```python
from build123d import *

# Parameters (mm, degrees)
SKETCH1_W           = 15.24
SKETCH1_H           = 44.45
SKETCH1_R           = 2.0193
SKETCH1_R_2         = 1.5
BOSS_EXTRUDE1_DEPTH = 3.429
FILLET1_R           = 2.54


with BuildPart() as part:
    # Sketch1 → Boss-Extrude1 (new body)
    with BuildSketch(Plane.XY):
        with Locations((0, 22.225)):
            Rectangle(SKETCH1_W, SKETCH1_H)
        with Locations((0, 4.445)):
            Circle(SKETCH1_R, mode=Mode.SUBTRACT)
        with Locations((0, 16.51)):
            Circle(SKETCH1_R, mode=Mode.SUBTRACT)
        with Locations((-5.08, 42.291)):
            Circle(SKETCH1_R_2, mode=Mode.SUBTRACT)
        with Locations((5.08, 42.291)):
            Circle(SKETCH1_R_2, mode=Mode.SUBTRACT)
    extrude(amount=BOSS_EXTRUDE1_DEPTH)

    # Fillet1
    fillet1_edges = [part.edges().sort_by_distance(p)[0] for p in [
        (7.62, 0, 1.7145),
        (-7.62, 0, 1.7145),
    ]]
    fillet(fillet1_edges, radius=FILLET1_R)


solid = part.part
```
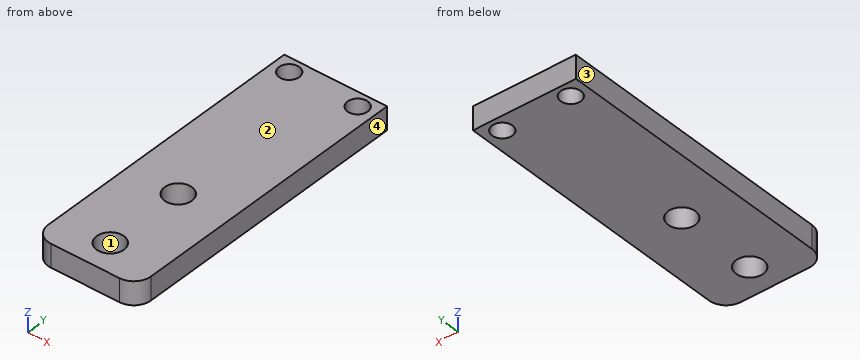
The listing builds one solid part. Answer for the finished solid, in the listing's coordinates (mm). Face numbers are marked on the shaded views. Coordinates: 2 decimals unless noted, no trailing zeros. Loops run counter-clockwise (first coordinate to the right, second up) from the corner with the lowest first, then second, coordinate; pieces in that order, holes last. Notation, with made-up numbers: (-22, 39.5) -> (-8, 39.5) arc R6 ccw to (-8, 50.5) -> close; hole circle Ø2 at (-33.75, -35). An arc over 180 degrees is marked (long way). Return JSON: item names as keys, results as strings. Group by question number.
(1) Find the intervals of material crossed by probe 1 along Y at (x, z) = (0, 1.15); probe 2 along Y at (x, z) = (-5.08, 2.1); probe 3 along Y at (x, z) = (1, 1.4), in increasing order. Write a range as from..to.
(2) A cutting plane is placed at B-B on x = 0. Write down the section's boundary in (y, z).
(3) A cutting plane is placed at A-A on y = 16.51. Write down the section's boundary in (x, z).
(4) A cutting plane is placed at C-C on x = 5.5. Write down the section's boundary in (y, z), and give its area (3 significant figures).
(5) Determine the mould class of the marked faces 1, 2, 3 and 4 for opening direction X: released by +X, released by -X, zero draft, split by the parting line, or undercut.
(6) A cutting plane is placed at D-D on z = 1.5. Write down the section's boundary in (x, y) (3 decimals).
The answers:
{
 "1": {"probe 1": "y = 0..2.43, 6.46..14.49, 18.53..44.45", "probe 2": "y = 0..40.79, 43.79..44.45", "probe 3": "y = 0..2.69, 6.2..14.76, 18.26..44.45"},
 "2": {"outline": "(0, 0) -> (2.43, 0) -> (2.43, 3.43) -> (0, 3.43) -> close; (6.46, 0) -> (14.49, 0) -> (14.49, 3.43) -> (6.46, 3.43) -> close; (18.53, 0) -> (44.45, 0) -> (44.45, 3.43) -> (18.53, 3.43) -> close"},
 "3": {"outline": "(-7.62, 0) -> (-2.02, 0) -> (-2.02, 3.43) -> (-7.62, 3.43) -> close; (2.02, 0) -> (7.62, 0) -> (7.62, 3.43) -> (2.02, 3.43) -> close"},
 "4": {"outline": "(0.03, 0) -> (40.85, 0) -> (40.85, 3.43) -> (0.03, 3.43) -> close; (43.73, 0) -> (44.45, 0) -> (44.45, 3.43) -> (43.73, 3.43) -> close", "area": "142 mm^2"},
 "5": {"face 1": "undercut", "face 2": "zero draft", "face 3": "released by -X", "face 4": "released by +X"},
 "6": {"outline": "(-7.62, 2.54) arc R2.54 ccw to (-5.08, 0) -> (5.08, 0) arc R2.54 ccw to (7.62, 2.54) -> (7.62, 44.45) -> (-7.62, 44.45) -> close; hole circle Ø3 at (-5.08, 42.291); hole circle Ø4.039 at (0, 4.445); hole circle Ø4.039 at (0, 16.51); hole circle Ø3 at (5.08, 42.291)"}
}
